Source: three-view drawing plus pictorial views. Frame: mm from the lowest corner of the part. A direction names the side the tool comes from. Give positions to 0.01 mm unless a question says otherwise; leave off trailing zeros. Order: outer loops, then holes, each group sorted by start corner. A loop starts at its lowest first (then second) coordinate and runs counter-clockwise, first axis right, second up. Notation, with made-up numbers: M -6,14 L 19,14 A22 ccw 19,23 Z; hole C -32.5,15.25 d10. An arc over 180 degrees is marked long. Use CSV: the item, a comma, the result in double quotes. Start each with the question number.
1. Section query D-D, the plane y = 31.5. Return the cut outline in (x, z).
2. Pin query (flat end, axial travel): P1, Ø1.6, axis at x = 14.5, z = 6.5, coming from the +Y side; P2, Ø3.5, axis at x = 12, y = 3, coming from the +Z side; P3, Ø10, axis at x = 6.5, y = 19, coming from the -Z side; P4, Ø1, axis at x = 16.5, z = 6.5, coming from the -Y side. Return the tip coordinate at first contact, or that it passes through.
3. Mould query, pull axis X, two halves, no side actions, for the marked faces 5, 6, 7 and 8. Classes: released by +X, released by -X, zero draft, split by the parting line, or undercut.
4. Line query: line 1 along Y through (x, z) = (13, 4) (1 decimal); line 2 along Y through (x, z) = (17.75, 8.25); line 3 along Z through (x, y) = (20.75, 19.05) (1 decimal). Output: solid intervals per line, ascending. Write a range as [from, to].
5. Reachability of the marked faces 1, 2, 3 and 4 from +Z, -Z, +X, -X, +Y, -Y: full face, straight path, thin tool, end or side. Return the list, or none.
6. Section query A-A, the plane x = 7. State how many separate pieces and enclosed holes the cut face has.
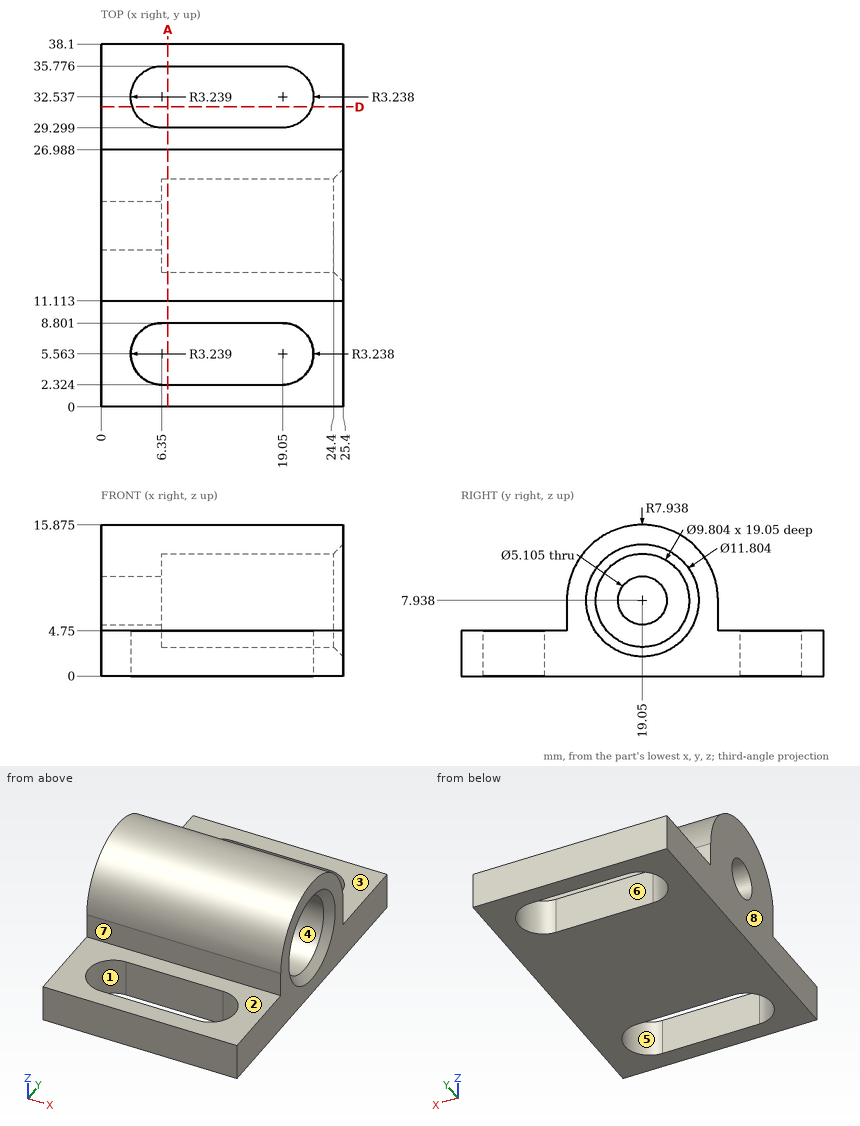
Result set:
1,outline,"M 0,0 L 3.28,0 L 3.28,4.75 L 0,4.75 Z; M 22.12,0 L 25.4,0 L 25.4,4.75 L 22.12,4.75 Z"
2,P1,"y = 26.99"
2,P2,"z = 4.75"
2,P3,"z = 0"
2,P4,"y = 11.11"
3,face 5,"undercut"
3,face 6,"undercut"
3,face 7,"zero draft"
3,face 8,"released by -X"
4,line 1,"[0, 2.3], [8.8, 16.1], [22, 29.3], [35.8, 38.1]"
4,line 2,"[11.12, 14.16], [23.94, 26.98]"
4,line 3,"[0, 3], [12.8, 15.9]"
5,face 1,"+Z, -Z"
5,face 2,"+Z, +X, -X, -Y"
5,face 3,"+Z, +X, -X, +Y"
5,face 4,"+X"
6,separate pieces,"3"
6,enclosed holes,"1"
